Autodesk Inventor part; units mm, degrees
ref_plane "YZ Plane" through (0, 0, 0) normal (1, 0, 0) x (0, 1, 0)
ref_plane "XZ Plane" through (0, 0, 0) normal (0, 1, 0) x (-1, 0, 0)
ref_plane "XY Plane" through (0, 0, 0) normal (0, 0, 1) x (1, 0, 0)
sketch "Sketch1" plane through (0, 0, 0) normal (0, 1, 0) x (-1, 0, 0)
  line L0 (0, -3.6919) -> (0, -9.1919)
  line L1 (0, -9.1919) -> (6, -9.1919)
  line L2 (0, -3.6919) -> (6, -3.6919)
  line L3 (6, -3.6919) -> (6, 3.0581)
  line L4 (6, 3.0581) -> (18, 3.0581)
  line L5 (18, 3.0581) -> (18, -15.9419)
  line L6 (18, -15.9419) -> (6, -15.9419)
  line L7 (6, -15.9419) -> (6, -9.1919)
  point P0 (0, 0)
  dimension "d0" = 5.5
  dimension "d1" = 6
  dimension "d3" = 12
  dimension "d4" = 6.75
  dimension "d5" = 6.75
  dimension "d6" = 19
  dimension "d7" = 12
sketch "Sketch2" plane through (0, 0, 0) normal (0, 1, 0) x (-1, 0, 0)
  point P0 (0, 0)
extrude "Extrusion1" add sketch "Sketch1" along normal blind 6
sketch "Sketch3" plane through (0, 6, 0) normal (0, 1, 0) x (1, 0, 0)
  line L0 (-6, 15.9419) -> (-18, 15.9419)
  line L1 (-6, -3.0581) -> (-6, 3.6919)
  line L2 (-18, 15.9419) -> (-6, 15.9419)
  line L3 (-6, 15.9419) -> (-6, -3.0581)
  line L4 (-6, -3.0581) -> (-18, -3.0581)
  line L5 (-18, -3.0581) -> (-18, 15.9419)
  point P0 (0, 0)
extrude "Extrusion2" cut sketch "Sketch3" against normal blind 2
sketch "Sketch4" plane through (-18, 0, -15.9419) normal (-1, 0, 0) x (0, 0, 1)
  point P0 (15.9419, 0)
sketch "Sketch5" plane through (-18, 0, 3.0581) normal (0, 0, 1) x (1, 0, 0)
  line L0 (12, 4) -> (0, 4)
  line L1 (0, 0) -> (12, 0)
  line L2 (12, 4) -> (0, 4)
  line L3 (0, 4) -> (0, 0)
  line L4 (0, 0) -> (12, 0)
  line L5 (12, 0) -> (12, 4)
  point P0 (18, 0)
extrude "Extrusion3" add sketch "Sketch5" along normal blind 2
sketch "Sketch6" plane through (-6, 0, -15.9419) normal (0, 0, -1) x (-1, 0, 0)
  line L0 (12, 4) -> (0, 4)
  line L1 (0, 0) -> (12, 0)
  line L2 (0, 4) -> (12, 4)
  line L3 (12, 4) -> (12, 0)
  line L4 (12, 0) -> (0, 0)
  line L5 (0, 0) -> (0, 4)
  point P0 (-6, 0)
extrude "Extrusion4" add sketch "Sketch6" along normal blind 2
sketch "Sketch7" plane through (-18, 0, 5.0581) normal (-1, 0, 0) x (0, 0, 1)
  point P0 (-5.0581, 0)
sketch "Sketch8" plane through (-18, 0, 5.0581) normal (-1, 0, 0) x (0, 0, 1)
  point P0 (-5.0581, 0)
sketch "Sketch9" plane through (0, 4, 0) normal (0, 1, 0) x (1, 0, 0)
  line L0 (-18, -5.0581) -> (-6, -5.0581)
  line L1 (-6, 9.1919) -> (-6, 17.9419)
  line L2 (-18, -5.0581) -> (-6, -5.0581)
  line L3 (-6, -5.0581) -> (-6, 17.9419)
  line L4 (-6, 17.9419) -> (-18, 17.9419)
  line L5 (-18, 17.9419) -> (-18, -5.0581)
  point P0 (0, 0)
extrude "Extrusion5" add sketch "Sketch9" along normal blind 1.5
sketch "Sketch10" plane through (-18, 0, -17.9419) normal (-1, 0, 0) x (0, 0, 1)
  line L0 (1.5, 1) -> (21.5, 1)
  line L1 (21.5, 1) -> (21.5, 4.5)
  line L2 (21.5, 4.5) -> (1.5, 4.5)
  line L3 (1.5, 4.5) -> (1.5, 1)
  line L4 (0, 5.5) -> (23, 5.5)
  line L5 (23, 0) -> (0, 0)
  line L6 (0, 0) -> (0, 5.5)
  line L7 (23, 0) -> (23, 5.5)
  point P0 (17.9419, 0)
  dimension "d22" = 1
  dimension "d23" = 1
  dimension "d24" = 1.5
  dimension "d25" = 1.5
extrude "Extrusion6" cut sketch "Sketch10" against normal blind 10 contours L3 L2 L1 L0
sketch "Sketch11" plane through (0, 0, -3.6919) normal (1, 0, 0) x (0, 0, -1)
  line L0 (14.25, 5.5) -> (-8.75, 5.5)
  line L1 (5, 5.5) -> (0.5, 5.5)
  line L2 (0.5, 5.5) -> (0.5, 0.5)
  line L3 (0.5, 0.5) -> (5, 0.5)
  line L4 (5, 0.5) -> (5, 5.5)
  line L5 (0, 0) -> (5.5, 0)
  line L6 (0, 0) -> (0, 6)
  line L7 (5.5, 0) -> (5.5, 6)
  point P0 (-3.6919, 0)
  point P1 (0.5, 5.5)
  dimension "d28" = 0.5
  dimension "d29" = 0.5
  dimension "d30" = 0.5
extrude "Extrusion7" cut sketch "Sketch11" against normal blind 6 contours L4 L3 L2 L0
sketch "Sketch12" plane through (0, 0, 0) normal (0, -1, 0) x (1, 0, 0)
  point P0 (0, 0)
sketch "Sketch13" plane through (0, 0, 0) normal (0, -1, 0) x (1, 0, 0)
  point P0 (0, 0)
sketch "Sketch14" plane through (0, 0, 0) normal (0, -1, 0) x (1, 0, 0)
  point P0 (0, 0)
sketch "Sketch15" plane through (0, 0, 0) normal (0, -1, 0) x (1, 0, 0)
  line L0 (-17.25, -11.9419) -> (-6.75, -11.9419)
  line L1 (-6.75, -11.9419) -> (-6.75, -0.9419)
  line L2 (-6.75, -0.9419) -> (-17.25, -0.9419)
  line L3 (-17.25, -0.9419) -> (-17.25, -11.9419)
  line L4 (-6, -17.9419) -> (-18, -17.9419)
  line L5 (-18, 5.0581) -> (-6, 5.0581)
  line L6 (-18, 5.0581) -> (-18, -17.9419)
  line L7 (-6, -3.6919) -> (-6, 5.0581)
  point P0 (0, 0)
  dimension "d33" = 6
  dimension "d34" = 6
  dimension "d35" = 0.75
  dimension "d36" = 0.75
extrude "Extrusion8" cut sketch "Sketch15" against normal up to surface (4.5 mm away)
properties part number "tof-mount"
The model under review builds one solid part; all positions refer to its coordinate system, in mm. A direction names the side the tool comes from. Round coordinates to 2 decimals unless told otherwise and drop trailing zeros. Loops run counter-clockwise (first coordinate to the right, second up) from the corner with the lowest first, then second, coordinate; pieces in that order, holes last. Notation, with made-up numbers: (-38, 12) -> (3, 12) arc R23 cw to (3, 38) -> close; hole circle Ø9 at (84, 78.25). An arc over 180 degrees is marked (long way). Write item = value, one per line. Start each with the question number.
Item 1: Take a section at B-B on x = -3.75. Give the boundary of the cut face in (y, z), plus the area to 3 significant figures.
Item 2: For faces 1 (the flat face through (-8, 3, -14)), 2 (the flat face through (-6, 3, -14)), 3 (the flat face through (-12, 5.5, -7)), 4 (the flat face through (-6, 3, 1)), 5 (the flat face through (-3, 3, -8.692)), list the 3-axis set-ups (+Z, -Z, +X, -X, +Y, -Y) from which the entire face can be reached by the end or side of a thin tool; tool diameter is ignored.
Item 3: To check wall thickness, follow L1, parallel to Y at x = -5, z = -5.5; L2, parallel to Z at x = -15.75, y = 1.6; L3, parallel to Z at x = -1.25, y = 0.95. State the ranges of each line that lie inside material, in increasing order.
Item 4: Take a section at C-C on z = -1.75. Give the boundary of the cut face in (x, y), plus the area to 3 significant figures.
Item 5: Insertion check: pin 1 (2 mm diameter, centred on y = 2.5, z = -5.5, fed in from +X); pin 2 (1.5 mm diameter, centred on x = -2, y = 4, fed in from -Z); pin 3 (3 mm diameter, centred on x = -13.5, z = -3, fed in from +Y). Each pin has a flat end and moves straight along its axis. Give the tip position at first contact, or say it passes through.
Item 6: Take a section at D-D on y = 5.2. Give the boundary of the cut face in (x, z).
Item 7: Mouldability with a two-part tool opening along Z and no side actions: class faces 6 (the flat face through (0, 3, -4)), 7 (the flat face through (-13, 3, 3.558)), 8 (the flat face through (-3, 3, -3.692)) as released by +Z, released by -Z, zero draft, split by the parting line, or undercut.
Result:
q1.outline = (0, -9.19) -> (6, -9.19) -> (6, -3.69) -> (0, -3.69) -> close; hole (0.5, -8.69) -> (5.5, -8.69) -> (5.5, -4.19) -> (0.5, -4.19) -> close
q1.area = 10.5 mm²
q2.face_1 = -X
q2.face_2 = -Z, +X, +Y, -Y
q2.face_3 = +Z, -Z, -X, +Y
q2.face_4 = +Z, +X, +Y, -Y
q2.face_5 = +X
q3.L1 = 0 to 0.5, 5.5 to 6
q3.L2 = -17.94 to -16.44, 3.56 to 5.06
q3.L3 = -9.19 to -8.69, -4.19 to -3.69
q4.outline = (-18, 0) -> (-17.25, 0) -> (-17.25, 1) -> (-18, 1) -> close; (-18, 4.5) -> (-6.75, 4.5) -> (-6.75, 0) -> (-6, 0) -> (-6, 5.5) -> (-18, 5.5) -> close
q4.area = 16.1 mm²
q5.pin_1 = -6
q5.pin_2 = -9.19
q5.pin_3 = 5.5
q6.outline = (-18, -17.94) -> (-6, -17.94) -> (-6, -9.19) -> (0, -9.19) -> (0, -8.69) -> (-6, -8.69) -> (-6, -4.19) -> (0, -4.19) -> (0, -3.69) -> (-6, -3.69) -> (-6, 5.06) -> (-18, 5.06) -> close
q7.face_6 = zero draft
q7.face_7 = undercut
q7.face_8 = released by +Z
